Input: part model. Units: mm. Frame: model coordinates. A direction names the side the tool comes from. Give positions to 0.01 mm unless a question says otherwise; leave off trailing zeros. Loops run counter-clockwise (first coordinate to the right, second up) from the corner with the lowest first, then second, coordinate; pieces in that order, holes last. Notation, with made-up numbers: M -14,-35.5 L 15,-35.5 A18 cw 15,-0.5 Z; hole C 36,64.25 d3. An arc over 180 degrees is marked long. One line per item, written item: value. Start each with the question number.
(1) Section D-D on z = -20. Output: boundary loops of the cut face in (x, y) (3 decimals).
(2) Section A-A on y = 87.5. Output: boundary loops of the cut face in (x, z) (3 decimals), plus the area to 3 significant figures.
(3) Access query for faces 1 (the cylindrical face through (44.79, 35.24, 2.17)), 2 (the cylindrical face through (0.97, 56.9, -21.98)), 3 (the flat face through (0, 15, 0)), 4 (the cylindrical face through (-54.918, 90.917, -20.759)). Directions: +Z, -Z, +X, -X, +Y, -Y. A direction counts if a zero-diameter tool reaches every point of the face in a straight line with its end or side. Return the directions, or none.
(4) Ray query, line 1 along Y through (x, z) = (38, 0); line 2 along Y through (x, z) = (-33, 0); line 3 along Z through (x, y) = (12.5, 65). Return the intervals inside material, ascending. Write a range as from..to.
(5) Section C-C on y = 67.5. Output: boundary loops of the cut face in (x, z) (3 decimals), plus the area to 3 significant figures.
(6) Pin query (flat end, axial travel): P1, Ø16, axis at x = -0.5, z = 1.5, coming from the +Y side; P2, Ø8, axis at x = 31.5, y = 47, coming from the +Z side; P3, Ø10, axis at y = 42.5, z = -16.5, coming from the -X side (3 decimals). Return the tip coordinate at first contact, or that it passes through.
(7) Section B-B on x = 20. Output: boundary loops of the cut face in (y, z), plus the area to 3 significant figures.
(8) Pull-direction query (X, two-part tool) for faces 5 (the cylindrical face through (-34.275, 99.423, 3.755)), 6 (the flat face through (-12.93, 100, 11.3)), 7 (the flat face through (-30, 7, 0)), 8 (the cylindrical face through (-30.42, 97.415, -1.302)); classes: released by +X, released by -X, zero draft, split by the parting line, or undercut.
```python
from build123d import *

# Parameters (mm, degrees)
SKETCH1_W                             = 60
SKETCH1_H                             = 60
BOSS_EXTRUDE1_DEPTH                   = 15
SKETCH2_R                             = 22
BOSS_EXTRUDE2_DEPTH                   = 85
SKETCH3_R                             = 17
BOSS_EXTRUDE3_DEPTH                   = 30
HOLE1_D                               = 20
HOLE1_DEPTH                           = 115
SKETCH9_R                             = 5
CUT_EXTRUDE1_DEPTH                    = 123.576506721
MIRROR2_COPY_1_SKETCH_R               = 5
MIRROR2_COPY_1_DEPTH                  = 123.576506721
BOSS_EXTRUDE4_REACH                   = 162.935
BOSS_EXTRUDE4_END_RADIUS              = 22
SKETCH10_R                            = 12.5
SKETCH11_R                            = 30
BOSS_EXTRUDE5_DEPTH                   = 10
HOLE2_REACH                           = 162.935
HOLE2_BORE_R                          = 10
TAP_DRILL_FOR_M8X1_0_TAP1_D           = 7
TAP_DRILL_FOR_M8X1_0_TAP1_DEPTH       = 10
TAP_DRILL_FOR_M8X1_0_TAP1_CSINK_D     = 7.05
TAP_DRILL_FOR_M8X1_0_TAP1_CSINK_ANGLE = 90
CIRPATTERN1_COUNT                     = 4
BOSS_EXTRUDE6_REACH                   = 211.444
BOSS_EXTRUDE6_END_RADIUS              = 22
BOSS_EXTRUDE6_START                   = -30
SKETCH18_R                            = 12.5
SKETCH20_R                            = 10
BOSS_EXTRUDE7_DEPTH                   = 30
HOLE3_REACH                           = 181.444
HOLE3_BORE_R                          = 6


with BuildPart() as part:
    # Sketch1 → Boss-Extrude1 (new body)
    with BuildSketch(Plane(origin=(0, 0, 0), x_dir=(1, 0, 0), z_dir=(0, 1, 0))):
        Rectangle(SKETCH1_W, SKETCH1_H)
    extrude(amount=BOSS_EXTRUDE1_DEPTH)

    # Sketch2 → Boss-Extrude2 (add)
    with BuildSketch(Plane(origin=(0, 15, 0), x_dir=(1, 0, 0), z_dir=(0, 1, 0))):
        with Locations(Location((0, 0, 0), (0, 0, 270))):
            Circle(SKETCH2_R)
    extrude(amount=BOSS_EXTRUDE2_DEPTH)

    # Sketch3 → Boss-Extrude3 (add)
    with BuildSketch(Plane(origin=(0, 100, 0), x_dir=(1, 0, 0), z_dir=(0, 1, 0))):
        with Locations(Location((0, 0, 0), (0, 0, 270))):
            Circle(SKETCH3_R)
    extrude(amount=BOSS_EXTRUDE3_DEPTH)

    # Hole1
    with Locations(Plane(origin=(0, 130, 0), x_dir=(1, 0, 0), z_dir=(0, 1, 0))):
        with Locations((0, 0)):
            Hole(HOLE1_D / 2, depth=HOLE1_DEPTH)

    # Sketch9 → Cut-Extrude1 (cut, through all)
    with BuildSketch(Plane(origin=(0, 15, 0), x_dir=(1, 0, 0), z_dir=(0, 1, 0))):
        with Locations(Location((20, 20, 0), (0, 0, 270))):
            Circle(SKETCH9_R)
    cut_extrude1 = extrude(amount=-CUT_EXTRUDE1_DEPTH, mode=Mode.SUBTRACT)

    # Mirror1: Cut-Extrude1 across plane
    add(cut_extrude1.mirror(Plane(origin=(0, 0, 0), x_dir=(0, 0, 1), z_dir=(1, 0, 0))), mode=Mode.SUBTRACT)

    # Mirror2: Cut-Extrude1 across plane
    add(cut_extrude1.mirror(Plane.XY), mode=Mode.SUBTRACT)

    # Mirror2 copy 1 sketch → Mirror2 copy 1 (cut, through all)
    with BuildSketch(Plane(origin=(0, 15, 0), x_dir=(-1, 0, 0), z_dir=(0, 1, 0))):
        with Locations(Location((20, 20, 0), (0, 0, 270))):
            Circle(MIRROR2_COPY_1_SKETCH_R)
    extrude(amount=-MIRROR2_COPY_1_DEPTH, mode=Mode.SUBTRACT)

    # Boss-Extrude4: up to this cylinder (the profile starts outside it)
    boss_extrude4_end = Plane(origin=(0, 87.5, 0), z_dir=(0, -1, 0)) * Cylinder(BOSS_EXTRUDE4_END_RADIUS, 370.87, mode=Mode.PRIVATE)
    # Sketch10 → Boss-Extrude4 (add, up to the surface)
    with BuildSketch(Plane(origin=(-60, 0, 0), x_dir=(0, 0, -1), z_dir=(1, 0, 0)), mode=Mode.PRIVATE) as boss_extrude4_sk1:
        with Locations(Location((0, 87.5, 0), (0, 0, 90))):
            Circle(SKETCH10_R)
    boss_extrude4_tool1 = extrude(boss_extrude4_sk1.sketch, amount=BOSS_EXTRUDE4_REACH, mode=Mode.PRIVATE) - boss_extrude4_end
    add(boss_extrude4_tool1.solids().sort_by_distance((-60, 87.5, 0))[0])

    # Sketch11 → Boss-Extrude5 (add)
    with BuildSketch(Plane.ZY.offset(60)):
        with Locations((0, 87.5)):
            Circle(SKETCH11_R)
    extrude(amount=-BOSS_EXTRUDE5_DEPTH)

    # Hole2 bore → Hole2 (cut, up to next)
    with BuildSketch(Plane.ZY.offset(60), mode=Mode.PRIVATE) as hole2_sk1:
        with Locations((0, 87.5)):
            Circle(HOLE2_BORE_R)
    hole2_tool1 = extrude(hole2_sk1.sketch, amount=-HOLE2_REACH, mode=Mode.PRIVATE) & part.part
    add(hole2_tool1.solids().sort_by_distance((-60, 87.5, 0))[0], mode=Mode.SUBTRACT)

    # Tap Drill for M8x1.0 Tap1
    with Locations(Plane.ZY.offset(60)):
        with Locations((20, 87.5)):
            tap_drill_for_m8x1_0_tap1 = CounterSinkHole(TAP_DRILL_FOR_M8X1_0_TAP1_D / 2, TAP_DRILL_FOR_M8X1_0_TAP1_CSINK_D / 2, depth=TAP_DRILL_FOR_M8X1_0_TAP1_DEPTH, counter_sink_angle=TAP_DRILL_FOR_M8X1_0_TAP1_CSINK_ANGLE)

    # CirPattern1: Tap Drill for M8x1.0 Tap1 ×4 about axis
    cirpattern1_axis = Axis((0, 87.5, 0), (1, 0, 0))
    for i in range(1, CIRPATTERN1_COUNT):
        add(tap_drill_for_m8x1_0_tap1.rotate(cirpattern1_axis, i * 360 / CIRPATTERN1_COUNT), mode=Mode.SUBTRACT)

    # Boss-Extrude6: up to this cylinder (the profile starts outside it)
    boss_extrude6_end = Plane(origin=(0, 45, 0), z_dir=(0, -1, 0)) * Cylinder(BOSS_EXTRUDE6_END_RADIUS, 467.888, mode=Mode.PRIVATE)
    # Sketch18 → Boss-Extrude6 (add, up to the surface)
    with BuildSketch(Plane(origin=(60, 0, 0), x_dir=(0, 0, -1), z_dir=(1, 0, 0)).offset(BOSS_EXTRUDE6_START), mode=Mode.PRIVATE) as boss_extrude6_sk1:
        with Locations((0, 45)):
            Circle(SKETCH18_R)
    boss_extrude6_tool1 = extrude(boss_extrude6_sk1.sketch, amount=-BOSS_EXTRUDE6_REACH, mode=Mode.PRIVATE) - boss_extrude6_end
    add(boss_extrude6_tool1.solids().sort_by_distance((30, 45, 0))[0])

    # Sketch20 → Boss-Extrude7 (add)
    with BuildSketch(Plane(origin=(30, 0, 0), x_dir=(0, 0, -1), z_dir=(1, 0, 0))):
        with Locations((0, 45)):
            Circle(SKETCH20_R)
    extrude(amount=BOSS_EXTRUDE7_DEPTH)

    # Hole3 bore → Hole3 (cut, up to next)
    with BuildSketch(Plane(origin=(60, 0, 0), x_dir=(0, 0, -1), z_dir=(1, 0, 0)), mode=Mode.PRIVATE) as hole3_sk1:
        with Locations((0, 45)):
            Circle(HOLE3_BORE_R)
    hole3_tool1 = extrude(hole3_sk1.sketch, amount=-HOLE3_REACH, mode=Mode.PRIVATE) & part.part
    add(hole3_tool1.solids().sort_by_distance((60, 45, 0))[0], mode=Mode.SUBTRACT)


solid = part.part
```
Output values:
1. outline: M -60,65.139 L -50,65.139 L -50,84 L -59.975,84 L -60,83.975 Z; M -60,91.025 L -59.975,91 L -50,91 L -50,109.861 L -60,109.861 Z; M -30,0 L -25,0 L -25,15 L -30,15 Z; M -15,0 L 15,0 L 15,15 L 9.165,15 L 9.165,100 L -9.165,100 L -9.165,15 L -15,15 Z; M 25,0 L 30,0 L 30,15 L 25,15 Z
2. outline: M -60,-30 L -50,-30 L -50,-23.5 L -59.975,-23.5 L -60,-23.525 Z; M -60,-16.475 L -59.975,-16.5 L -50,-16.5 L -50,-12.5 L -18.104,-12.5 A22 ccw long -18.104,12.5 L -50,12.5 L -50,16.5 L -59.975,16.5 L -60,16.475 L -60,10 L 0,10 A10 cw 0,-10 L -60,-10 Z; M -60,23.525 L -59.975,23.5 L -50,23.5 L -50,30 L -60,30 Z
2. area: 1,350 mm²
3. face 1: +X
3. face 2: none
3. face 3: +Y
3. face 4: -X
4. line 1: y = 35..39, 51..55
4. line 2: y = 75..77.5, 97.5..100
4. line 3: z = -18.1..18.1
5. outline: M -60,-22.361 L -50,-22.361 L -50,-3.5 L -59.975,-3.5 L -60,-3.525 Z; M -60,3.525 L -59.975,3.5 L -50,3.5 L -50,22.361 L -60,22.361 Z; C 0,0 d44; hole C 0,0 d20
5. area: 1,580 mm²
6. P1: stops at y = 15
6. P2: stops at z = 12.5
6. P3: stops at x = -18.755
7. outline: M 0,-30 L 15,-30 L 15,-25 L 0,-25 Z; M 0,-15 L 15,-15 L 15,-9.17 L 36.5,-9.17 A12.5 ccw 53.5,-9.17 L 100,-9.17 L 100,9.17 L 53.5,9.17 A12.5 ccw 36.5,9.17 L 15,9.17 L 15,15 L 0,15 Z; M 0,25 L 15,25 L 15,30 L 0,30 Z; hole C 45,0 d12
7. area: 2,120 mm²
8. face 5: undercut
8. face 6: undercut
8. face 7: released by -X
8. face 8: zero draft
